from build123d import *

# Parameters (mm, degrees)
SKETCH1_W           = 41.91
SKETCH1_H           = 19.05
BOSS_EXTRUDE1_DEPTH = 2.54
SKETCH1_3_W         = 41.91
SKETCH1_3_H         = 19.05
BOSS_EXTRUDE2_DEPTH = 30.48


with BuildPart() as part:
    # Sketch1 → Boss-Extrude1 (new body)
    with BuildSketch(Plane.XY):
        Polygon((0, 42.164), (0, 0), (41.91, 0), (41.91, 19.05), (83.82, 19.05), (83.82, 0), (104.648, 0), (104.648, 19.05), (146.558, 19.05), (146.558, 0), (190.5, 0), (190.5, 42.164), align=None)
        with Locations((62.865, 9.525)):
            Rectangle(SKETCH1_W, SKETCH1_H)
        with Locations((125.603, 9.525)):
            Rectangle(SKETCH1_W, SKETCH1_H)
    extrude(amount=-BOSS_EXTRUDE1_DEPTH)

    # Sketch1_3 → Boss-Extrude2 (add)
    with BuildSketch(Plane.XY):
        with Locations((62.865, 9.525)):
            Rectangle(SKETCH1_3_W, SKETCH1_3_H)
        with Locations((125.603, 9.525)):
            Rectangle(SKETCH1_3_W, SKETCH1_3_H)
    extrude(amount=BOSS_EXTRUDE2_DEPTH)


solid = part.part
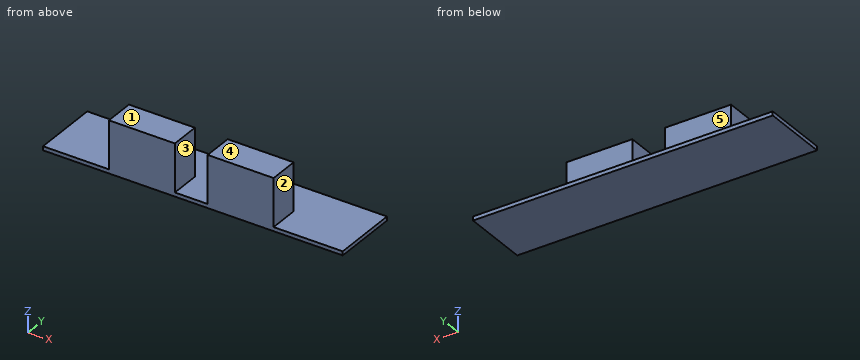
For this review, take the finished solid that the model builds, in its own axes (mm). Face numbers are marked on the shaded views. A direction names the side the tool comes from. Round coordinates to 2 decimals unless told otherwise and drop trailing zeros. Write each loop counter-clockwise with the first axis right and the second up, starting at its lowest first coordinate (ties: lowest second). Pieces come first, ordered by that corner, then holes. Notation, with made-up numbers: (-25.75, -17.75) -> (17.25, -17.75) arc R22 cw to (17.25, 6.25) -> close; hole circle Ø1 at (-38, 85). An arc over 180 degrees is marked (long way). Use CSV: the item, a comma, the result in double quotes.
(1) Consider section B-B, the plane y = 12. Give the boundary of the cut face in (x, z), plus the area to 3 significant figures.
Computed values:
outline,"(0, -2.54) -> (190.5, -2.54) -> (190.5, 0) -> (146.56, 0) -> (146.56, 30.48) -> (104.65, 30.48) -> (104.65, 0) -> (83.82, 0) -> (83.82, 30.48) -> (41.91, 30.48) -> (41.91, 0) -> (0, 0) -> close"
area,"3,040 mm²"
(2) Clearance check with flat-ended pins moving along their axes: P1, Ø12, axis at y = 10, z = 14, coming from the -X side; P2, Ø4, axis at x = 82, z = 17.5, coming from the +Y side; P3, Ø8, axis at x = 31.5, z = 5.5, coming from the -Y side. State where each tip first meets the part, or that it passes through.
Computed values:
P1,"x = 41.91"
P2,"y = 19.05"
P3,"through"
(3) Consider section D-D, the plane y = 39.5. Give the boundary of the cut face in (x, z), plus the area to 3 significant figures.
Computed values:
outline,"(0, -2.54) -> (190.5, -2.54) -> (190.5, 0) -> (0, 0) -> close"
area,"484 mm²"
(4) For the marked faces 4 and 5, list the 3-axis set-ups (+Z, -Z, +X, -X, +Y, -Y) from which the entire face can be reached by the end or side of a thin tool; tool diameter is ignored.
Computed values:
face 4,"+Z, +X, -X, +Y, -Y"
face 5,"+Z, +X, -X, +Y"
(5) To check wall thickness, follow L1, parallel to X at y = 8, z = 12.5; L2, parallel to Z at x = 131, y = 22; L3, parallel to Y at x = 79.5, z = 5.5. State the ranges of each line that lie inside material, in increasing order. Write a range as [from, to].
Computed values:
L1,"[41.91, 83.82], [104.65, 146.56]"
L2,"[-2.54, 0]"
L3,"[0, 19.05]"
(6) Draft analysis for pull direction X (two halves, no side actions). For the marked faces 1, 2 and 3, state which applies: +X half, -X half, draft (parallel to the pull), parting line (faces both ways), or undercut.
Computed values:
face 1,"draft"
face 2,"+X half"
face 3,"undercut"
(7) Consider section A-A, the plane z = 14.5. Give the boundary of the cut face in (x, y).
Computed values:
outline,"(41.91, 0) -> (83.82, 0) -> (83.82, 19.05) -> (41.91, 19.05) -> close; (104.65, 0) -> (146.56, 0) -> (146.56, 19.05) -> (104.65, 19.05) -> close"
(8) Consider section C-C, the plane x = 125. Give the boundary of the cut face in (y, z), plus the area to 3 significant figures.
Computed values:
outline,"(0, -2.54) -> (42.16, -2.54) -> (42.16, 0) -> (19.05, 0) -> (19.05, 30.48) -> (0, 30.48) -> close"
area,"688 mm²"
